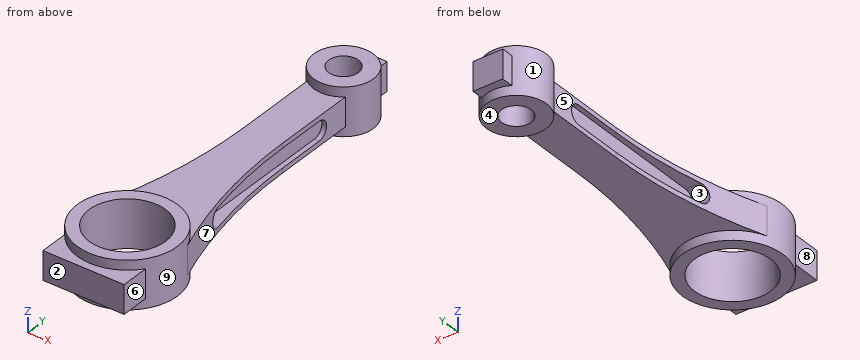
from build123d import *

# Parameters (mm, degrees)
SKETCH2_R             = 21
SKETCH2_R_2           = 16
BOSS_EXTRUDE1_DEPTH   = 10
SKETCH2_R_3           = 12.5
SKETCH2_R_4           = 6.25
BOSS_EXTRUDE1_2_DEPTH = 10
BOSS_EXTRUDE2_DEPTH   = 6
BOSS_EXTRUDE3_DEPTH   = 6
CUT_EXTRUDE1_DEPTH    = 62


with BuildPart() as part:
    # Sketch2 → Boss-Extrude1 (new, symmetric)
    with BuildSketch(Plane.XY):
        Circle(SKETCH2_R)
        Circle(SKETCH2_R_2, mode=Mode.SUBTRACT)
    extrude(amount=BOSS_EXTRUDE1_DEPTH, both=True)



with BuildPart() as body_2:
    # Sketch2 → Boss-Extrude1 2 (new, symmetric)
    with BuildSketch(Plane.XY):
        with Locations((0, 120)):
            Circle(SKETCH2_R_3)
        with Locations((0, 120)):
            Circle(SKETCH2_R_4, mode=Mode.SUBTRACT)
    extrude(amount=BOSS_EXTRUDE1_2_DEPTH, both=True)


with BuildPart() as part_1:
    add(part.part)

    add(body_2.part)  # Boss-Extrude2 merges body 2
    # Sketch3 → Boss-Extrude2 (add, symmetric)
    with BuildSketch(Plane.XY):
        with BuildLine():
            Line((-8, 110.395313644), (-8, 75.395313644))
            ThreePointArc((-8, 75.395313644), (-10.96842855, 40.709642053), (-19.787382488, 7.032744434))
            ThreePointArc((-19.787382488, 7.032744434), (0, 21), (19.787382488, 7.032744434))
            ThreePointArc((19.787382488, 7.032744434), (10.96842855, 40.709642053), (8, 75.395313644))
            Line((8, 75.395313644), (8, 110.395313644))
            ThreePointArc((8, 110.395313644), (0, 107.5), (-8, 110.395313644))
        make_face()
    extrude(amount=BOSS_EXTRUDE2_DEPTH, both=True)

    # Sketch4 → Boss-Extrude3 (add, symmetric)
    with BuildSketch(Plane.XY):
        with BuildLine():
            Line((0, 132.5), (0, 135.825317547))
            Line((0, 135.825317547), (-6.25, 135.825317547))
            Line((-6.25, 135.825317547), (-6.25, 130.825317547))
            ThreePointArc((-6.25, 130.825317547), (-3.235238064, 132.074072829), (0, 132.5))
        make_face()
        with BuildLine():
            Line((6.25, 135.825317547), (0, 135.825317547))
            Line((0, 135.825317547), (0, 132.5))
            ThreePointArc((0, 132.5), (3.235238064, 132.074072829), (6.25, 130.825317547))
            Line((6.25, 130.825317547), (6.25, 135.825317547))
        make_face()
        with BuildLine():
            ThreePointArc((-17, -12.328828006), (0, -21), (17, -12.328828006))
            Line((17, -12.328828006), (17, -24.328828006))
            Line((17, -24.328828006), (-17, -24.328828006))
            Line((-17, -24.328828006), (-17, -12.328828006))
        make_face()
    extrude(amount=BOSS_EXTRUDE3_DEPTH, both=True)

    # Sketch5 → Cut-Extrude1 (cut)
    with BuildSketch(Plane(origin=(6, 0, 0), x_dir=(0, 0, -1), z_dir=(1, 0, 0))):
        with BuildLine():
            Line((4, 96), (4, 34))
            ThreePointArc((4, 34), (0, 30), (-4, 34))
            Line((-4, 34), (-4, 96))
            ThreePointArc((-4, 96), (0, 100), (4, 96))
        make_face()
    cut_extrude1 = extrude(amount=CUT_EXTRUDE1_DEPTH, mode=Mode.SUBTRACT)

    # Mirror1: Cut-Extrude1 across plane
    add(cut_extrude1.mirror(Plane(origin=(0, 0, 0), x_dir=(0, 0, 1), z_dir=(1, 0, 0))), mode=Mode.SUBTRACT)


solid = part_1.part
Source: CAD feature listing. Evaluate the final solid. Frame: model axes, mm. Face numbers are marked on the shaded views. A direction names the side the tool comes from. Round coordinates to 2 decimals unless told otherwise and drop trailing zeros. Loops run counter-clockwise (first coordinate to the right, second up) from the corner with the lowest first, then second, coordinate; pieces in that order, holes last.
Q1. Access query for the marked faces 5, 6, 7, 8 and 9. Directions: +Z, -Z, +X, -X, +Y, -Y. A direction counts if a zero-diameter tool reaches every point of the face in a straight line with its end or side. Return the directions, or none.
Q2. Section C-C, the plane y = 0. Return loops of the section in (x, z).
Q3. First-contact query: P1, Ø1.5, axis at y = 132.5, z = -3, coming from the -X side; P2, Ø2.5, axis at y = 55.5, z = 1, coming from the +X side; P3, Ø8, axis at x = -8, y = 41.5, coming from the -Z side; P4, Ø6, axis at x = 12.5, y = 86, coming from the +Z side. Flat tips, straight axial feed; report the tip coordinate or a pass-through.
Q4. Section D-D, the plane z = 8.25. Return loops of the section in (x, y).
Q5. Section B-B, the plane z = 0. Return loops of the section in (x, y).
Q6. Section A-A, the plane x = 0. Return loops of the section in (y, z), plus the area to 3 significant figures.
Q7. Ray query, line 1 (Y direction, x = 0, z = -1.5); line 2 (Y direction, x = -4, z = -4.25); line 3 (Y direction, x = -1.5, z = -7.75). Return the intervals inside material, ascending.
Q8. Mould query, pull axis Y, two halves, no side actions, for the marked faces 1, 2, 3 and 4. Classes: pulls with the +Y half, pulls with the -Y half, needs draft (parallel to the pull), parting line crosses it, or undercut.
Solutions:
1. face 5: +Z, -Z, -X
1. face 6: +Z, -Z, +X, -Y
1. face 7: +Z, -Z, +X
1. face 8: +Z, -Z, -X, -Y
1. face 9: none
2. outline: (-21, -10) - (-16, -10) - (-16, 10) - (-21, 10) - close; (16, -10) - (21, -10) - (21, 10) - (16, 10) - close
3. P1: stops at x = -6.25
3. P2: stops at x = 6
3. P3: stops at z = -6
3. P4: passes through
4. outline: circle Ø42 at (0, 0); circle Ø25 at (0, 120); hole circle Ø32 at (0, 0); hole circle Ø12.5 at (0, 120)
5. outline: (-19.79, 7.03) arc R21 ccw to (-17, -12.33) - (-17, -24.33) - (17, -24.33) - (17, -12.33) arc R21 ccw to (19.79, 7.03) arc R204.13 cw to (13.11, 30) - (6, 30) - (6, 100) - (8, 100) - (8, 110.4) arc R12.5 ccw to (6.25, 130.83) - (6.25, 135.83) - (-6.25, 135.83) - (-6.25, 130.83) arc R12.5 ccw to (-8, 110.4) - (-8, 100) - (-6, 100) - (-6, 30) - (-13.11, 30) arc R204.13 cw to start; hole circle Ø32 at (0, 0); hole circle Ø12.5 at (0, 120)
6. outline: (-24.33, -6) - (-21, -6) - (-21, -10) - (-16, -10) - (-16, 10) - (-21, 10) - (-21, 6) - (-24.33, 6) - close; (16, -10) - (21, -10) - (21, -6) - (107.5, -6) - (107.5, -10) - (113.75, -10) - (113.75, 10) - (107.5, 10) - (107.5, 6) - (21, 6) - (21, 10) - (16, 10) - close; (126.25, -10) - (132.5, -10) - (132.5, -6) - (135.83, -6) - (135.83, 6) - (132.5, 6) - (132.5, 10) - (126.25, 10) - close
6. area: 1,570 mm2
7. line 1: y = -24.33 to -16, 16 to 113.75, 126.25 to 135.83
7. line 2: y = -24.33 to -15.49, 15.49 to 115.2, 124.8 to 135.83
7. line 3: y = -20.95 to -15.93, 15.93 to 20.95, 107.59 to 113.93, 126.07 to 132.41
8. face 1: undercut
8. face 2: pulls with the -Y half
8. face 3: undercut
8. face 4: needs draft
